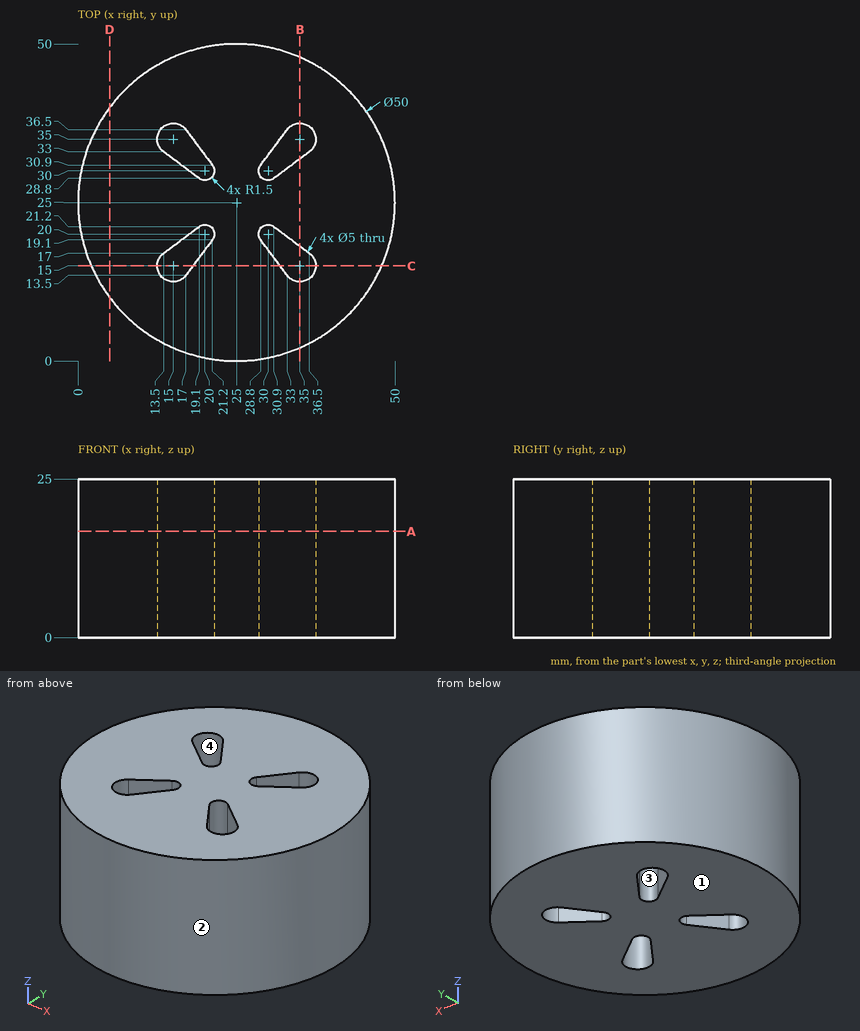
For this review, use the dimensioned drawing (mm, ordinates from the lowest corner) and the shaded views. Give positions to 0.01 mm unless a question says otherwise; leave off trailing zeros. Write each loop counter-clockwise with the first axis right and the second up, starting at its lowest first coordinate (ties: lowest second). Pieces come first, ordered by that corner, then holes. Notation, with made-up numbers: M -31.75,8.25 L 8.25,8.25 A16 ccw 8.25,14.25 Z; hole C 74,84 d7. An arc over 180 degrees is marked long. Answer as a JSON object with one key per item and string values. Group by question number.
Item 1: For probe 1 along X at (y, z) = (35, 10.25) (3 decimals); probe 2 along X at (y, z) = (30.5, 2), list the stretches that pass through material, from the lowest coordinate up. Write a range as [from, to].
Item 2: Consider section D-D on x = 5. Write out the cut boundary in (y, z).
Item 3: For pin 1 Ø10 at (x, z) = (11.5, 4) entering from +Y; pin 2 Ø4 at (y, z) = (27, 20) entering from -X; pin 3 Ø1.5 at (x, z) = (17, 3) entering from -Y; pin 4 Ø12 at (x, z) = (23.5, 11.5) entering from -Y, all flat-tipped, find the tip position at first contact; note any pin that passes through.
Item 4: Consider section A-A on z = 16.75. Write out the cut boundary in (x, y), plus the area to 3 significant figures.
Item 5: Consider section B-B on x = 35. Write out the cut boundary in (y, z) (3 decimals), plus the area to 3 significant figures.
Item 6: Draft analysis for pull direction X (two halves, no side actions). For the marked faces 1, 2, 3 and 4, state which applies: +X half, -X half, draft (parallel to the pull), parting line (faces both ways), or undercut.
Check result:
{
 "1": {"probe 1": "x = [2.087, 12.5], [18.125, 31.875], [37.5, 47.913]", "probe 2": "x = [0.61, 16.83], [21.41, 28.59], [33.17, 49.39]"},
 "2": {"outline": "M 10,0 L 40,0 L 40,25 L 10,25 Z"},
 "3": {"pin 1": "stops at y = 48.51", "pin 2": "stops at x = 0", "pin 3": "stops at y = 1.07", "pin 4": "stops at y = 0"},
 "4": {"outline": "C 25,25 d50; hole M 13.5,17 A2.5 ccw long 17,13.5 L 21.2,19.1 A1.5 ccw 19.1,21.2 Z; hole M 13.5,33 L 19.1,28.8 A1.5 ccw 21.2,30.9 L 17,36.5 A2.5 ccw long Z; hole M 28.8,19.1 L 33,13.5 A2.5 ccw long 36.5,17 L 30.9,21.2 A1.5 ccw Z; hole M 28.8,30.9 A1.5 ccw 30.9,28.8 L 36.5,33 A2.5 ccw long 33,36.5 Z", "area": "1,800 mm^2"},
 "5": {"outline": "M 2.087,0 L 12.5,0 L 12.5,25 L 2.087,25 Z; M 18.125,0 L 31.875,0 L 31.875,25 L 18.125,25 Z; M 37.5,0 L 47.913,0 L 47.913,25 L 37.5,25 Z", "area": "864 mm^2"},
 "6": {"face 1": "draft", "face 2": "parting line", "face 3": "undercut", "face 4": "undercut"}
}
